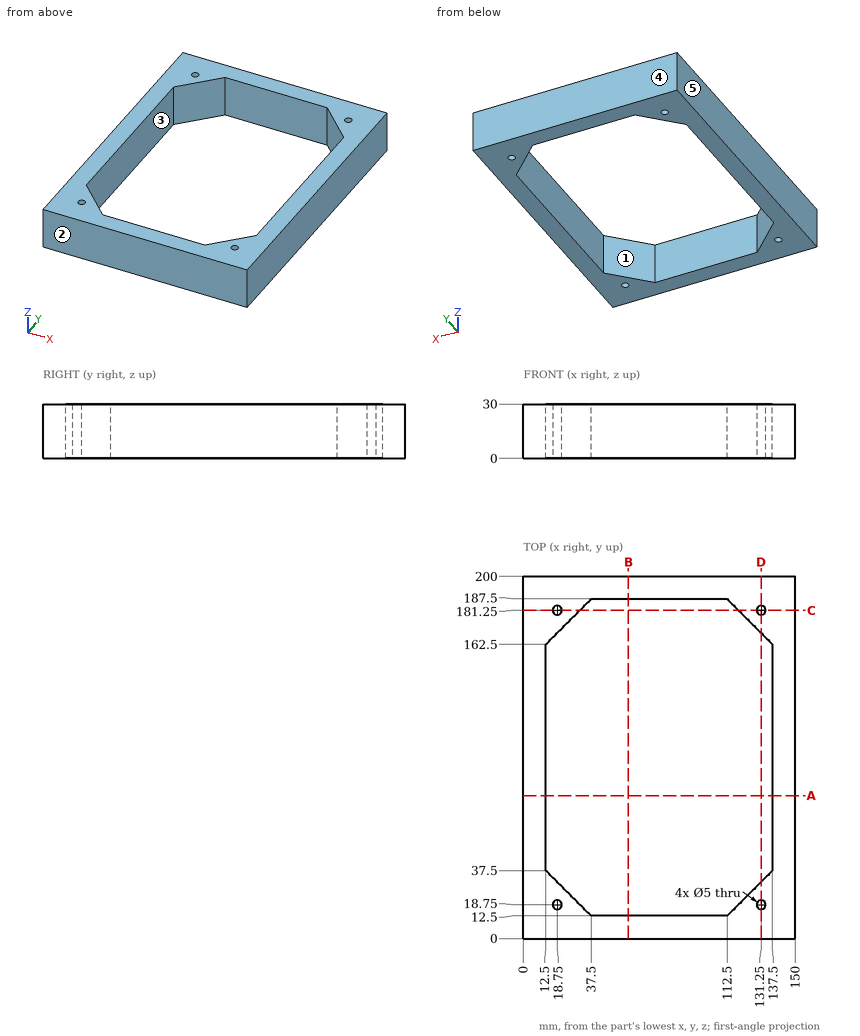
Design review of the part shown in the three views and the two pictorial views. Dimensions are in mm from the part's minimum x, y and z. A direction names the side the tool comes from. Round coordinates to 2 decimals unless told otherwise and drop trailing zeros. Loops run counter-clockwise (first coordinate to the right, second up) from the corner with the lowest first, then second, coordinate; pieces in that order, holes last.
Q1. Insertion check: pin 1 Ø1 at (x, z) = (123, 3.5) entering from -Y. The pin has a flat end and moves straight along its axis. Give the tip position at first contact, or say it passes through.
Result sheet:
pin 1: stops at y = 0
Q2. Add section D-D on x = 131.25. Write out the cut boundary in (y, z), plus the area to 4 significant figures.
Result sheet:
outline: (0, 0) - (16.25, 0) - (16.25, 30) - (0, 30) - close; (21.25, 0) - (31.25, 0) - (31.25, 30) - (21.25, 30) - close; (168.75, 0) - (178.75, 0) - (178.75, 30) - (168.75, 30) - close; (183.75, 0) - (200, 0) - (200, 30) - (183.75, 30) - close
area: 1,575 mm2
Q3. Add section C-C on y = 181.25. Write out the cut boundary in (x, z).
Result sheet:
outline: (0, 0) - (16.25, 0) - (16.25, 30) - (0, 30) - close; (21.25, 0) - (31.25, 0) - (31.25, 30) - (21.25, 30) - close; (118.75, 0) - (128.75, 0) - (128.75, 30) - (118.75, 30) - close; (133.75, 0) - (150, 0) - (150, 30) - (133.75, 30) - close
Q4. Machinability: for the marked faces 1 and 2, which of the approach directions +Z, -Z, +X, -X, +Y, -Y give a long, thin tool a straight path to every point of the face, cutting with its end or side? Answer none if there is none.
Result sheet:
face 1: +Z, -Z
face 2: +Z, -Z, +X, -X, -Y
Q5. To check wall thickness, follow line 1 along X through (y, z) = (123, 15.25); line 2 along Y through (x, z) = (18.75, 9.5); line 3 along Y through (x, z) = (60, 21.25). State the ranges of each line that lie inside material, in increasing order.
Result sheet:
line 1: x = 0 to 12.5, 137.5 to 150
line 2: y = 0 to 16.25, 21.25 to 31.25, 168.75 to 178.75, 183.75 to 200
line 3: y = 0 to 12.5, 187.5 to 200
Q6. Add section A-A on y = 79. Write out the cut boundary in (x, z).
Result sheet:
outline: (0, 0) - (12.5, 0) - (12.5, 30) - (0, 30) - close; (137.5, 0) - (150, 0) - (150, 30) - (137.5, 30) - close
Q7. Mouldability with a two-part tool opening along Y and no side actions: class the marked faces 3, 4 and 5 as +Y half, -Y half, draft (parallel to the pull), parting line (faces both ways), or undercut.
Result sheet:
face 3: undercut
face 4: +Y half
face 5: draft
Q8. Add section B-B on x = 58. Write out the cut boundary in (y, z).
Result sheet:
outline: (0, 0) - (12.5, 0) - (12.5, 30) - (0, 30) - close; (187.5, 0) - (200, 0) - (200, 30) - (187.5, 30) - close
